Autodesk Inventor part; units mm, degrees
ref_plane "XZ Plane" through (0, 0, 0) normal (0, 1, 0) x (-1, 0, 0)
ref_plane "XY Plane" through (0, 0, 0) normal (0, 0, 1) x (1, 0, 0)
sketch "Sketch1" plane through (0, 0, 0) normal (0, 0, 1) x (1, 0, 0)
  line L0 (-12.7, -25.4) -> (12.7, -25.4)
  line L1 (12.7, -25.4) -> (12.7, 25.4)
  line L2 (12.7, 25.4) -> (-12.7, 25.4)
  line L3 (-12.7, 25.4) -> (-12.7, -25.4)
  line L4 (-12.7, -25.4) -> (12.7, 25.4) construction
  line L5 (12.7, -25.4) -> (-12.7, 25.4) construction
  line L6 (-9.525, 22.225) -> (9.525, 22.225)
  line L7 (9.525, 22.225) -> (9.525, -22.225)
  line L8 (9.525, -22.225) -> (-9.525, -22.225)
  line L9 (-9.525, -22.225) -> (-9.525, 22.225)
  point P0 (0, 0)
  dimension "width" = 25.4
  dimension "height" = 50.8
  dimension "thickness" = 3.175
extrude "Extrusion1" add sketch "Sketch1" along normal mid plane 254
sketch "Sketch2" plane through (12.7, -25.4, 127) normal (1, 0, 0) x (0, 0, -1)
  line L0 (254, 50.8) -> (254, 0) construction
  line L1 (254, 0) -> (0, 0) construction
  line L2 (0, 0) -> (0, 50.8) construction
  line L3 (0, 50.8) -> (254, 50.8) construction
  circle A0 centre (31.75, 25.4) radius 23.8125 construction
  circle A1 centre (31.75, 25.4) radius 25.4 construction
  point P0 (127, 25.4)
  point P1 (57.15, 25.4)
  point P2 (53.747, 38.1)
  point P3 (44.45, 47.397)
  point P4 (31.75, 50.8)
  point P5 (19.05, 47.397)
  point P6 (9.753, 38.1)
  point P7 (6.35, 25.4)
  point P8 (9.753, 12.7)
  point P9 (19.05, 3.403)
  point P10 (31.75, 0)
  point P11 (44.45, 3.403)
  point P12 (53.747, 12.7)
  point P13 (55.5625, 25.4)
  point P14 (43.6562, 46.0222)
  point P15 (19.8437, 46.0222)
  point P16 (7.9375, 25.4)
  point P17 (19.8437, 4.7778)
  point P18 (43.6562, 4.7778)
  dimension "d13" = 47.625
  dimension "d14" = 50.8
  dimension "d5" = 31.75
  dimension "d17" = 360
  dimension "d21" = 360
hole "Hole1" at (12.7, 0, 95.25) direction (-1, 0, 0) diameter 28.956 end through all
hole "Hole2" at (12.7, 12.7, 73.253) at (12.7, 0, 69.85) at (12.7, -12.7, 73.253) at (12.7, -12.7, 117.247) at (12.7, 0, 120.65) at (12.7, 12.7, 117.247) direction (-1, 0, 0) diameter 5.1054 end through all
hole "Hole3" at (12.7, -20.6222, 107.1562) at (12.7, -20.6222, 83.3438) at (12.7, 0, 119.0625) at (12.7, 20.6222, 107.1562) at (12.7, 20.6222, 83.3438) at (12.7, 0, 71.4375) direction (-1, 0, 0) diameter 4.4958 end through all
sketch "Sketch3" plane through (-12.7, 25.4, 127) normal (0, 1, 0) x (1, 0, 0)
  line L0 (0, 0) -> (25.4, 0) construction
  line L1 (6.096, 0) -> (19.304, 0)
  line L2 (19.304, 0) -> (19.304, 38.1)
  line L3 (19.304, 38.1) -> (6.096, 38.1)
  line L4 (6.096, 38.1) -> (6.096, 0)
  line L5 (25.4, 0) -> (0, 0) construction
  point P0 (12.7, 127)
  point P1 (12.7, 38.1)
  point P2 (12.7, 0)
  dimension "d37" = 13.208
  dimension "d38" = 38.1
extrude "Extrusion2" cut sketch "Sketch3" against normal through all
properties part number "CL4-001" material "Aluminum 6061"
Input: part model. Units: mm. Frame: model coordinates. A direction names the side the tool comes from. Round coordinates to 2 decimals unless told otherwise and drop trailing zeros. Loops run counter-clockwise (first coordinate to the right, second up) from the corner with the lowest first, then second, coordinate; pieces in that order, holes last.
1) Material intervals for line 1 (X direction, y = -21.5, z = 63) (3 decimals); line 2 (Y direction, x = 1.75, z = -21) (3 decimals); line 3 (Z direction, x = 11.4, y = -12.7), sorted ascending.
Ans:
line 1: x = -12.7 to -9.525, 9.525 to 12.7
line 2: y = -25.4 to -22.225, 22.225 to 25.4
line 3: z = -127 to 70.7, 75.81 to 88.3, 102.2 to 114.69, 119.8 to 127
2) Pull-direction query (Y, two-part tool) for faces 1 (the flat face through (0, 25.4, -2)), 2 (the cylindrical face through (-0.18, -22.85, 83.64)), 3 (the flat face through (12.7, 0, -2)); classes: released by +Y, released by -Y, zero draft, split by the parting line, or undercut.
Ans:
face 1: released by +Y
face 2: undercut
face 3: zero draft
3) Set-up query: faces 4 (the flat face through (9.525, 0, -2)), 5 (the flat face through (-11, 0, 127)). Return all of +Z, -Z, +X, -X, +Y, -Y with unobstructed straight access to the full face (end or side cutting, diameter ignored); none if empty.
Ans:
face 4: +Z, -Z
face 5: +Z, +X, -X, +Y, -Y
4) Pin query (flat end, axial travel): pin 1 (10 mm diameter, centred on x = 5.5, y = -6, fed in from +Z); pin 2 (3.5 mm diameter, centred on x = 0.5, y = 23.5, fed in from +Z). Return the tip coordinate at first contact, or that it passes through.
Ans:
pin 1: stops at z = 127
pin 2: stops at z = 88.9
5) Section query A-A on x = 2. Return the cut outline in (y, z) (3 decimals), plus the area to 3 significant figures.
Ans:
outline: (-25.4, -127) - (-22.225, -127) - (-22.225, 81.768) arc R2.248 cw to (-22.225, 84.92) - (-22.225, 88.9) - (-25.4, 88.9) - close; (22.225, -127) - (25.4, -127) - (25.4, 88.9) - (22.225, 88.9) - (22.225, 84.92) arc R2.248 cw to (22.225, 81.768) - close
area: 1,370 mm2
6) Section query D-D on z = 100. Return the cut outline in (x, y) (3 decimals), plus the area to 3 significant figures.
Ans:
outline: (-12.7, -25.4) - (-6.604, -25.4) - (-6.604, -22.225) - (-9.525, -22.225) - (-9.525, -13.677) - (-12.7, -13.677) - close; (-12.7, 13.677) - (-9.525, 13.677) - (-9.525, 22.225) - (-6.604, 22.225) - (-6.604, 25.4) - (-12.7, 25.4) - close; (6.604, -25.4) - (12.7, -25.4) - (12.7, -13.677) - (9.525, -13.677) - (9.525, -22.225) - (6.604, -22.225) - close; (6.604, 22.225) - (9.525, 22.225) - (9.525, 13.677) - (12.7, 13.677) - (12.7, 25.4) - (6.604, 25.4) - close
area: 186 mm2
7) Section query B-B on z = 33. Return the cut outline in (x, y) (3 decimals).
Ans:
outline: (-12.7, -25.4) - (12.7, -25.4) - (12.7, 25.4) - (-12.7, 25.4) - close; hole (-9.525, -22.225) - (9.525, -22.225) - (9.525, 22.225) - (-9.525, 22.225) - close
8) Section query C-C on y = 0. Count the separate pieces of the cut face and the enclosed holes in it, plus the area to 3 significant figures.
Ans:
separate pieces: 8
enclosed holes: 0
area: 1,350 mm2
